from build123d import *

# Parameters (mm, degrees)
F0_W     = 39
F0_H     = 10
F1_DEPTH = 110
F2_W     = 35
F2_H     = 1
F3_DEPTH = 110
F5_DEPTH = 110
F6_W     = 22
F6_H     = 12
F7_DEPTH = 110
F8_R     = 2.1
F9_DEPTH = 25
F10_SIZE = 0.2
F11_R    = 0.5


with BuildPart() as f1:
    # F0 (on Right) → F1 (new body)
    with BuildSketch(Plane.YZ):
        Rectangle(F0_W, F0_H)
    extrude(amount=F1_DEPTH)

    # F2 (on face) → F3 (cut)
    with BuildSketch(Plane.YZ.offset(110)):
        with Locations((0, 5)):
            Rectangle(F2_W, F2_H)
    extrude(amount=-F3_DEPTH, mode=Mode.SUBTRACT)

    # F4 (on face) → F5 (cut)
    with BuildSketch(Plane.YZ.offset(110)):
        Polygon((-18.5, 3), (18.5, 3), (18.5, 4.5), (17.5, 4.5), (17.5, 5.544198), (-17.5, 5.544198), (-17.5, 4.5), (-18.5, 4.5), align=None)
    extrude(amount=-F5_DEPTH, mode=Mode.SUBTRACT)

    # F6 (on face) → F7 (cut)
    with BuildSketch(Plane.YZ.offset(110)):
        with Locations((0, 3)):
            Rectangle(F6_W, F6_H)
    extrude(amount=-F7_DEPTH, mode=Mode.SUBTRACT)

    # F8 (on face) → F9 (cut)
    with BuildSketch(Plane.XY.offset(-3)):
        with Locations((15, 0)):
            Circle(F8_R)
        with Locations((95, 0)):
            Circle(F8_R)
        with Locations((55, -7.5)):
            Circle(F8_R)
        with Locations((55, 7.5)):
            Circle(F8_R)
    extrude(amount=-F9_DEPTH, mode=Mode.SUBTRACT)

    # F10
    f10_edges = [f1.edges().sort_by_distance(p)[0] for p in [
        (55, -19.5, 5),
        (55, 19.5, 5),
    ]]
    chamfer(f10_edges, length=F10_SIZE)

    # F11
    f11_edges = [f1.edges().sort_by_distance(p)[0] for p in [
        (0, -19.5, -0.1),
        (0, 19.5, -0.1),
        (110, -19.5, -0.1),
        (110, 19.5, -0.1),
    ]]
    fillet(f11_edges, radius=F11_R)


solid = f1.part
Read the model definition and answer for the solid it produces. Units are mm, in the model's axes. A direction names the side the tool comes from. Give positions to 0.01 mm unless a question says otherwise; leave off trailing zeros. Loops run counter-clockwise (first coordinate to the right, second up) from the corner with the lowest first, then second, coordinate; pieces in that order, holes last. Notation, with made-up numbers: M 12.25,-28.75 L 40.25,-28.75 A23 cw 40.25,-5.75 Z; hole C -31.75,81.5 d11. An arc over 180 degrees is marked long. Write each question's results on one line, items separated by ' | '.
1. Section D-D on y = 13 is taken. Give the vertices of the cut face in (x, z), plus the area to 3 significant figures.
Values:
outline: M 0,-5 L 110,-5 L 110,3 L 0,3 Z | area: 880 mm^2
2. Section B-B on y = 0 is taken. Give the vertices of the cut face in (x, z), plus the area to 3 significant figures.
Values:
outline: M 0,-5 L 12.9,-5 L 12.9,-3 L 0,-3 Z; M 17.1,-5 L 92.9,-5 L 92.9,-3 L 17.1,-3 Z; M 97.1,-5 L 110,-5 L 110,-3 L 97.1,-3 Z | area: 203 mm^2
3. Section A-A on x = 55 is taken. Give the vertices of the cut face in (y, z).
Values:
outline: M -19.5,-5 L -9.6,-5 L -9.6,-3 L -11,-3 L -11,3 L -18.5,3 L -18.5,4.5 L -17.5,4.5 L -17.5,5 L -19.3,5 L -19.5,4.8 Z; M -5.4,-5 L 5.4,-5 L 5.4,-3 L -5.4,-3 Z; M 9.6,-5 L 19.5,-5 L 19.5,4.8 L 19.3,5 L 17.5,5 L 17.5,4.5 L 18.5,4.5 L 18.5,3 L 11,3 L 11,-3 L 9.6,-3 Z
4. Straight lines are drawn through the part: line 1 (Y direction, x = 102, z = -2.5); line 2 (Y direction, x = 15, z = -3.5); line 3 (Z direction, x = 37, y = -18). For each, find the intervals that lie inside material, in ascending order. Write a range as [from, to].
Values:
line 1: y = [-19.5, -11], [11, 19.5] | line 2: y = [-19.5, -2.1], [2.1, 19.5] | line 3: z = [-5, 3], [4.5, 5]
5. A tool of negligible diameter and unlimited length cuts with its end or side. For faces 4 (the face through (56, -11, 0)), 5 (the face through (92.9, 0.09, -3.99)), from which of +Z, -Z, +X, -X, +Y, -Y can it reach the whole face along a straight path? Write none if from no direction.
Values:
face 4: +Z, +X, -X | face 5: +Z, -Z
6. The mould has two halves that part along Y. Classify faces 1 (the face through (110, -0.3, -3.3)), 2 (the face through (12.9, 0.09, -3.99)), 3 (the face through (54, -19.5, 0)): pulls with the +Y half, pulls with the -Y half, needs draft (parallel to the pull), parting line crosses it, or undercut.
Values:
face 1: needs draft | face 2: undercut | face 3: pulls with the -Y half
7. Section C-C on x = 95 is taken. Give the vertices of the cut face in (y, z), plus the area to 3 significant figures.
Values:
outline: M -19.5,-5 L -2.1,-5 L -2.1,-3 L -11,-3 L -11,3 L -18.5,3 L -18.5,4.5 L -17.5,4.5 L -17.5,5 L -19.3,5 L -19.5,4.8 Z; M 2.1,-5 L 19.5,-5 L 19.5,4.8 L 19.3,5 L 17.5,5 L 17.5,4.5 L 18.5,4.5 L 18.5,3 L 11,3 L 11,-3 L 2.1,-3 Z | area: 177 mm^2
8. Given pin 1 (5.5 mm diameter, centred on x = 55, y = 7.5, fed in from +Z); pin 2 (4 mm diameter, centred on x = 52, y = 13.5, fed in from +Z), each flat-ended and moving along its own axis, determine where each tip first touches the part or whether it passes through.
Values:
pin 1: stops at z = -3 | pin 2: stops at z = 3
